from build123d import *

# Parameters (mm, degrees)
SKETCH_1_W          = 12.7
SKETCH_1_H          = 5.08
EXTRUDE_1_DEPTH     = 8.89
SKETCH_2_R          = 0.762
EXTRUDE_2_DEPTH     = 1.778
SKETCH_3_R          = 0.762
EXTRUDE_3_DEPTH     = 2.032
FILLET_2_R          = 1
FILLET_3_R          = 1
SKETCH_4_R          = 1.143
CUT_EXTRUDE_1_DEPTH = 6


with BuildPart() as part:
    # Эскиз1 → Бобышка-Вытянуть1 (new body)
    with BuildSketch(Plane.XY):
        Rectangle(SKETCH_1_W, SKETCH_1_H)
    extrude(amount=EXTRUDE_1_DEPTH)

    # Эскиз2 → Бобышка-Вытянуть2 (add)
    with BuildSketch(Plane(origin=(0, 0, 0), x_dir=(-1, 0, 0), z_dir=(0, 0, -1))):
        with Locations(Location((-4.7498, 0, 0), (0, 0, 180))):
            Circle(SKETCH_2_R)
        with Locations(Location((0, 0, 0), (0, 0, 180))):
            Circle(SKETCH_2_R)
        with Locations(Location((4.7498, 0, 0), (0, 0, 180))):
            Circle(SKETCH_2_R)
    extrude(amount=EXTRUDE_2_DEPTH)

    # Эскиз3 → Бобышка-Вытянуть3 (add)
    with BuildSketch(Plane.XY.offset(8.89)):
        with Locations((-2.3876, 0)):
            Circle(SKETCH_3_R)
    extrude(amount=EXTRUDE_3_DEPTH)

    # Скругление2
    fillet_2_edges = [part.edges().sort_by_distance(p)[0] for p in [
        (-6.35, 0, 8.89),
        (0, -2.54, 8.89),
        (6.35, 0, 8.89),
        (0, 2.54, 8.89),
    ]]
    fillet(fillet_2_edges, radius=FILLET_2_R)

    # Скругление3
    # the kernel refuses this fillet: 1 mm, written as the material it takes off along each edge
    with BuildSketch(Plane(origin=(5.35, 1.54, 7.89), x_dir=(1, 0, 0), z_dir=(0, 1, 0))) as fillet_3_piece_1_section:
        Polygon((0, 0), (FILLET_3_R, 0), (FILLET_3_R, -FILLET_3_R), (0, -FILLET_3_R), align=None)
    fillet_3_piece_1 = extrude(amount=FILLET_3_R, mode=Mode.PRIVATE)
    fillet_3_piece_1 = fillet_3_piece_1 - Plane(origin=(5.35, 1.54, 7.89), x_dir=(-0.7071067811865475, 0, -0.7071067811865475), z_dir=(0, 1, 0)) * Sphere(FILLET_3_R, mode=Mode.PRIVATE)
    add(fillet_3_piece_1, mode=Mode.SUBTRACT)
    with BuildSketch(Plane(origin=(5.35, -1.54, 7.89), x_dir=(0, -1, 0), z_dir=(1, 0, 0))) as fillet_3_piece_2_section:
        Polygon((0, 0), (FILLET_3_R, 0), (FILLET_3_R, -FILLET_3_R), (0, -FILLET_3_R), align=None)
    fillet_3_piece_2 = extrude(amount=FILLET_3_R, mode=Mode.PRIVATE)
    fillet_3_piece_2 = fillet_3_piece_2 - Plane(origin=(5.35, -1.54, 7.89), x_dir=(0, 0.7071067811865475, -0.7071067811865475), z_dir=(1, 0, 0)) * Sphere(FILLET_3_R, mode=Mode.PRIVATE)
    add(fillet_3_piece_2, mode=Mode.SUBTRACT)
    with BuildSketch(Plane(origin=(-5.35, 1.54, 7.89), x_dir=(-1, 0, 0), z_dir=(0, 1, 0))) as fillet_3_piece_3_section:
        Polygon((0, 0), (FILLET_3_R, 0), (FILLET_3_R, FILLET_3_R), (0, FILLET_3_R), align=None)
    fillet_3_piece_3 = extrude(amount=FILLET_3_R, mode=Mode.PRIVATE)
    fillet_3_piece_3 = fillet_3_piece_3 - Plane(origin=(-5.35, 1.54, 7.89), x_dir=(0.7071067811865475, 0, -0.7071067811865475), z_dir=(0, 1, 0)) * Sphere(FILLET_3_R, mode=Mode.PRIVATE)
    add(fillet_3_piece_3, mode=Mode.SUBTRACT)
    with BuildSketch(Plane(origin=(-5.35, -1.54, 7.89), x_dir=(0, -1, 0), z_dir=(-1, 0, 0))) as fillet_3_piece_4_section:
        Polygon((0, 0), (FILLET_3_R, 0), (FILLET_3_R, FILLET_3_R), (0, FILLET_3_R), align=None)
    fillet_3_piece_4 = extrude(amount=FILLET_3_R, mode=Mode.PRIVATE)
    fillet_3_piece_4 = fillet_3_piece_4 - Plane(origin=(-5.35, -1.54, 7.89), x_dir=(0, 0.7071067811865475, -0.7071067811865475), z_dir=(-1, 0, 0)) * Sphere(FILLET_3_R, mode=Mode.PRIVATE)
    add(fillet_3_piece_4, mode=Mode.SUBTRACT)
    with BuildSketch(Plane(origin=(-6.35, -2.54, -2.5), x_dir=(0, 1, 0), z_dir=(0, 0, 1)), Plane(origin=(-6.35, 2.54, -2.5), x_dir=(1, 0, 0), z_dir=(0, 0, 1))) as fillet_3_piece_5:
        with BuildLine():
            CenterArc((FILLET_3_R, -FILLET_3_R), FILLET_3_R, 90, 90)
            Line((0, -FILLET_3_R), (0, 0))
            Line((0, 0), (FILLET_3_R, 0))
        make_face()
    extrude(amount=10.39, mode=Mode.SUBTRACT)
    with BuildSketch(Plane(origin=(6.35, -2.54, -2.5), x_dir=(0, 1, 0), z_dir=(0, 0, 1)), Plane(origin=(6.35, 2.54, -2.5), x_dir=(-1, 0, 0), z_dir=(0, 0, 1))) as fillet_3_piece_6:
        with BuildLine():
            CenterArc((FILLET_3_R, FILLET_3_R), FILLET_3_R, 180, 90)
            Line((0, FILLET_3_R), (0, 0))
            Line((0, 0), (FILLET_3_R, 0))
        make_face()
    extrude(amount=10.39, mode=Mode.SUBTRACT)

    # Эскиз4 → Вырез-Вытянуть1 (cut)
    with BuildSketch(Plane(origin=(0, 2.54, 0), x_dir=(1, 0, 0), z_dir=(0, 1, 0))):
        with Locations(Location((-2.3876, -2.286, 0), (0, 0, 270))):
            Circle(SKETCH_4_R)
        with Locations(Location((2.3876, -2.286, 0), (0, 0, 270))):
            Circle(SKETCH_4_R)
    extrude(amount=-CUT_EXTRUDE_1_DEPTH, mode=Mode.SUBTRACT)


solid = part.part
For this review, take the finished solid that the model builds, in its own axes (mm). A direction names the side the tool comes from. Give positions to 0.01 mm unless a question says otherwise; leave off trailing zeros. Order: outer loops, then holes, each group sorted by start corner. A loop starts at its lowest first (then second) coordinate and runs counter-clockwise, first axis right, second up. Notation, with made-up numbers: M 46,-19.75 L 83,-19.75 A7 ccw 83,-15.75 Z; hole C 19.5,-26 d3. An arc over 180 degrees is marked long. Answer in a Markdown table with one row per item. Add a question column.
(1) Consider section C-C on z = -1. State the section outline as (x, y) points.
(2) Mouldability with a two-part tool opening along X and no side actions: class faces 1 (the face through (3.16, 0.036, 1.444)), 2 (the face through (6.1, 2.2, 3.9)), 3 (the face through (0, -2.54, 4)) as +X half, -X half, draft (parallel to the pull), parting line (faces both ways), or undercut.
(3) Consider section A-A on y = 0. State the section outline as (x, z) points, and give its area (3 significant figures).
(4) Consider section D-D on x = 1.5. State the section outline as (y, z) points, and give its area (3 significant figures).
(5) Wall thickness on probe 1 along Z at (x, y) = (-4.25, -0.1); probe 2 along X at (y, z) = (-2.2, 2.75); probe 3 along Z at (x, y) = (2.5, -0.1): over which ranges is each line inside the solid? List them lowest first. Write a range as [from, to].
(6) Consider section B-B on x = 3.75. State the section outline as (y, z) points, and give its area (3 significant figures).
(7) For faces 4 (the face through (-2, 0, 10.922)), 5 (the face through (-1.978, 0.643, 9.892)), 6 (the face through (5.477, -0.229, -0.877)), list the 3-axis set-ups (+Z, -Z, +X, -X, +Y, -Y) from which the entire face can be reached by the end or side of a thin tool; tool diameter is ignored.
Evaluation:
| question | item | result |
|---|---|---|
| 1 | outline | C -4.75,0 d1.52; C 0,0 d1.52; C 4.75,0 d1.52 |
| 2 | face 1 | undercut |
| 2 | face 2 | +X half |
| 2 | face 3 | draft |
| 3 | outline | M -6.35,0 L -5.51,0 L -5.51,-1.78 L -3.99,-1.78 L -3.99,0 L -0.76,0 L -0.76,-1.78 L 0.76,-1.78 L 0.76,0 L 3.99,0 L 3.99,-1.78 L 5.51,-1.78 L 5.51,0 L 6.35,0 L 6.35,7.89 A1 ccw 5.35,8.89 L -1.63,8.89 L -1.63,10.92 L -3.15,10.92 L -3.15,8.89 L -5.35,8.89 A1 ccw -6.35,7.89 Z; hole C -2.39,2.29 d2.29; hole C 2.39,2.29 d2.29 |
| 3 | area | 115 mm^2 |
| 4 | outline | M -2.54,0 L 2.54,0 L 2.54,1.57 L -2.54,1.57 Z; M -2.54,3.01 L 2.54,3.01 L 2.54,7.89 A1 ccw 1.54,8.89 L -1.54,8.89 A1 ccw -2.54,7.89 Z |
| 4 | area | 37.4 mm^2 |
| 5 | probe 1 | z = [-1.78, 8.89] |
| 5 | probe 2 | x = [-6.1, -3.43], [-1.34, 1.34], [3.43, 6.1] |
| 5 | probe 3 | z = [0, 1.15], [3.42, 8.89] |
| 6 | outline | M -2.54,0 L 2.54,0 L 2.54,7.89 A1 ccw 1.54,8.89 L -1.54,8.89 A1 ccw -2.54,7.89 Z |
| 6 | area | 44.7 mm^2 |
| 7 | face 4 | +Z, +X, -X, +Y, -Y |
| 7 | face 5 | +Z |
| 7 | face 6 | -Z |
